```python
from build123d import *

# Parameters (mm, degrees)
F0_R      = 12.7
F1_DEPTH  = 35.56
F2_R      = 7.62
F2_R_2    = 2.54
F3_DEPTH  = 10.16
F3_FACE_R = 2.54
F4_DEPTH  = 30.48


with BuildPart() as f1:
    # F0 (on Top) → F1 (new body)
    with BuildSketch(Plane.XY):
        Circle(F0_R)
    extrude(amount=F1_DEPTH)

    # F2 (on face) → F3 (cut)
    with BuildSketch(Plane.XY.offset(35.56)):
        Circle(F2_R)
        Circle(F2_R_2, mode=Mode.SUBTRACT)
    extrude(amount=-F3_DEPTH, mode=Mode.SUBTRACT)

    # F3_face (on face) → F4 (cut)
    with BuildSketch(Plane.XY.offset(35.56)):
        Circle(F3_FACE_R)
    extrude(amount=-F4_DEPTH, mode=Mode.SUBTRACT)


solid = f1.part
```
The model under review builds one solid part; all positions refer to its coordinate system, in mm. A direction names the side the tool comes from. Round coordinates to 2 decimals unless told otherwise and drop trailing zeros. Order: outer loops, then holes, each group sorted by start corner. A loop starts at its lowest first (then second) coordinate and runs counter-clockwise, first axis right, second up. Notation, with made-up numbers: (53, 46) -> (70, 46) arc R11 ccw to (70, 67) -> close; hole circle Ø2 at (23.5, 64). An arc over 180 degrees is marked (long way). One line per item, written item: value. Start each with the question number.
Q1. Machinability: for faces 4 (the face through (-1.65, -7.44, 30.55)), 5 (the face through (0, 0, 0)), which of the approach directions +Z, -Z, +X, -X, +Y, -Y give a long, thin tool a straight path to every point of the face, cutting with its end or side? Answer none if there is none.
Q2. Wall thickness on line 1 (Y direction, x = 0, z = 29); line 2 (Z direction, x = -2.75, y = 0.5); line 3 (X direction, y = 1.25, z = 13.5): over which ranges is each line inside the solid? List them lowest first.
Q3. Take a section at C-C (z = 21). Write out the cut boundary in (x, y).
Q4. Clearance check with flat-ended pins moving along their axes: pin 1 Ø5.5 at (x, y) = (-0.5, 1) entering from +Z; pin 2 Ø4 at (x, z) = (2.5, 5) entering from -Y; pin 3 Ø2 at (x, z) = (2.5, 30.5) entering from +Y. State where each tip first meets the part, or that it passes through.
Q5. Take a section at D-D (z = 29). Write out the cut boundary in (x, y), and give its area (3 significant figures).
Q6. Mouldability with a two-part tool opening along Y and no side actions: class faces 1 (the face through (5.5, -5.5, 35.56)), 2 (the face through (-2.75, -12.4, 17.53)), 3 (the face through (-0.33, 2.52, 15.38)) as released by +Y, released by -Y, zero draft, split by the parting line, or undercut.
Q7. Take a section at A-A (y = 0). Write out the cut boundary in (x, z), and give its area (3 significant figures).
Reported:
1. face 4: +Z
1. face 5: -Z, +X, -X, +Y, -Y
2. line 1: y = -12.7 to -7.62, 7.62 to 12.7
2. line 2: z = 0 to 25.4
2. line 3: x = -12.64 to -2.21, 2.21 to 12.64
3. outline: circle Ø25.4 at (0, 0); hole circle Ø5.08 at (0, 0)
4. pin 1: stops at z = 25.4
4. pin 2: stops at y = -12.69
4. pin 3: stops at y = 12.61
5. outline: circle Ø25.4 at (0, 0); hole circle Ø15.24 at (0, 0)
5. area: 324 mm2
6. face 1: zero draft
6. face 2: split by the parting line
6. face 3: undercut
7. outline: (-12.7, 0) -> (12.7, 0) -> (12.7, 35.56) -> (7.62, 35.56) -> (7.62, 25.4) -> (2.54, 25.4) -> (2.54, 5.08) -> (-2.54, 5.08) -> (-2.54, 25.4) -> (-7.62, 25.4) -> (-7.62, 35.56) -> (-12.7, 35.56) -> close
7. area: 645 mm2
